from build123d import *

# Parameters (mm, degrees)
F0_W           = 8.4991231561
F0_H           = 6.35
F1_DEPTH       = 12.7
F2_DEPTH       = 16.525
F3_DEPTH       = 7
F5_D           = 3.4544
F5_DEPTH       = 12.7
F5_CSINK_D     = 4.5974
F5_CSINK_ANGLE = 82
F5_TIP         = 1.0378064612


# Not quite as in the source:
# - a length typed as a fraction of an inch, garbled in the dataset ("3 / 203.2 mm" for 3/8 in), is restored


with BuildPart() as f1:
    # F0 (on Right) → F1 (new body)
    with BuildSketch(Plane.YZ):
        with BuildLine():
            ThreePointArc((19.0844833851, -6.525), (17.2246114456, -2.0348719395), (12.7344833851, -0.175))
            Line((12.7344833851, -0.175), (8.4991231561, -0.175))
            Line((8.4991231561, -0.175), (8.4991231561, -6.525))
            Line((8.4991231561, -6.525), (19.0844833851, -6.525))
        make_face()
        with BuildLine():
            Line((-8.4991231561, -0.175), (-12.7344833851, -0.175))
            ThreePointArc((-12.7344833851, -0.175), (-17.2246114456, -2.0348719395), (-19.0844833851, -6.525))
            Line((-19.0844833851, -6.525), (-8.4991231561, -6.525))
            Line((-8.4991231561, -6.525), (-8.4991231561, -0.175))
        make_face()
        with BuildLine():
            ThreePointArc((8.4901041675, 7.0058502143), (0, 3), (-8.4901041675, 7.0058502143))
            Line((-8.4901041675, 7.0058502143), (-12.7344833851, -0.175))
            Line((-12.7344833851, -0.175), (-8.4991231561, -0.175))
            Line((-8.4991231561, -0.175), (0, -0.175))
            Line((0, -0.175), (8.4991231561, -0.175))
            Line((8.4991231561, -0.175), (12.7344833851, -0.175))
            Line((12.7344833851, -0.175), (8.4901041675, 7.0058502143))
        make_face()
        with BuildLine():
            Line((-3.2282481135, 15.9081179517), (-8.4901041675, 7.0058502143))
            ThreePointArc((-8.4901041675, 7.0058502143), (0, 3), (8.4901041675, 7.0058502143))
            Line((8.4901041675, 7.0058502143), (3.2282481135, 15.9081179517))
            ThreePointArc((3.2282481135, 15.9081179517), (3.6172109716, 14.9890828009), (3.75, 14))
            ThreePointArc((3.75, 14), (-0.9890828009, 10.3827890284), (-3.2282481135, 15.9081179517))
        make_face()
        with BuildLine():
            ThreePointArc((3.2282481135, 15.9081179517), (0, 17.75), (-3.2282481135, 15.9081179517))
            ThreePointArc((-3.2282481135, 15.9081179517), (-0.9890828009, 10.3827890284), (3.75, 14))
            ThreePointArc((3.75, 14), (3.6172109716, 14.9890828009), (3.2282481135, 15.9081179517))
        make_face()
        with Locations((4.249561578, -3.35)):
            Rectangle(F0_W, F0_H)
        with Locations((-4.249561578, -3.35)):
            Rectangle(F0_W, F0_H)
    extrude(amount=F1_DEPTH)

    # F0 (on Right) → F2 (join)
    with BuildSketch(Plane.YZ):
        with BuildLine():
            ThreePointArc((3.2282481135, 15.9081179517), (0, 17.75), (-3.2282481135, 15.9081179517))
            ThreePointArc((-3.2282481135, 15.9081179517), (-0.9890828009, 10.3827890284), (3.75, 14))
            ThreePointArc((3.75, 14), (3.6172109716, 14.9890828009), (3.2282481135, 15.9081179517))
        make_face()
    extrude(amount=-F2_DEPTH)

    # F0 (on Right) → F3 (join)
    with BuildSketch(Plane.YZ):
        with BuildLine():
            ThreePointArc((19.0844833851, -6.525), (17.2246114456, -2.0348719395), (12.7344833851, -0.175))
            Line((12.7344833851, -0.175), (8.4991231561, -0.175))
            Line((8.4991231561, -0.175), (8.4991231561, -6.525))
            Line((8.4991231561, -6.525), (19.0844833851, -6.525))
        make_face()
        with BuildLine():
            Line((-8.4991231561, -0.175), (-12.7344833851, -0.175))
            ThreePointArc((-12.7344833851, -0.175), (-17.2246114456, -2.0348719395), (-19.0844833851, -6.525))
            Line((-19.0844833851, -6.525), (-8.4991231561, -6.525))
            Line((-8.4991231561, -6.525), (-8.4991231561, -0.175))
        make_face()
        with Locations((4.249561578, -3.35)):
            Rectangle(F0_W, F0_H)
        with Locations((-4.249561578, -3.35)):
            Rectangle(F0_W, F0_H)
    extrude(amount=-F3_DEPTH)

    # F5
    with Locations(Plane(origin=(0, 0, -6.525), x_dir=(1, 0, 0), z_dir=(0, 0, -1))):
        with Locations((6.35, 0)):
            CounterSinkHole(F5_D / 2, F5_CSINK_D / 2, depth=F5_DEPTH, counter_sink_angle=F5_CSINK_ANGLE)
            with Locations((0, 0, -(F5_DEPTH + F5_TIP / 2))):  # 118° drill point
                Cone(0, F5_D / 2, F5_TIP, mode=Mode.SUBTRACT)


solid = f1.part
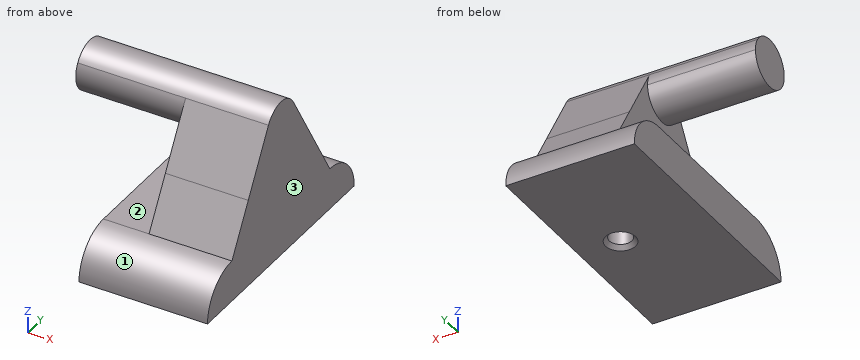
Geometry check sheet. Reference: the model listing, model coordinates, mm. Face numbers are marked on the shaded views. Round coordinates to 2 decimals unless told otherwise and drop trailing zeros. Order: outer loops, then holes, each group sorted by start corner. A loop starts at its lowest first (then second) coordinate and runs counter-clockwise, first axis right, second up. Notation, with made-up numbers: (7.5, 50) - (64.5, 50) arc R21 ccw to (64.5, 89) - close; hole circle Ø1 at (46.25, 88). An arc over 180 degrees is marked (long way). One line per question, with ' | ' between items. Start each with the question number.
(1) Release check for a two-part mould opening along Z. For the marked faces 1, 2 and 3 record: released by +Z, released by -Z, zero draft, split by the parting line, or undercut.
(2) Sectioned sample at B-B on z = 5. Record the cut outline in (x, y).
(3) Sectioned sample at C-C on y = 7.5. Record the cut outline in (x, z) (3 decimals), and give its area (3 significant figures).
(4) Depth check by flat-ended pin: pin 1 Ø1.9 at (y, z) = (-4.5, -2.5) entering from -X; pin 2 Ø5.5 at (x, y) = (-2.5, 5.5) entering from +Z; pin 3 Ø1 at (x, z) = (-11, 12) entering from +Y; pin 4 Ø5 at (x, z) = (-4.5, 6) entering from -Y. Enter the tip coordinate at first touch or a pass-through.
(5) Sectioned sample at A-A on x = 0.5. Record the cut outline in (y, z) (3 decimals).
(6) Thickness scan on L1, parallel to X at y = 6.5, z = 5.5; L2, parallel to X at y = -13, z = -3.75; L3, parallel to Y at x = 7.25, z = -1.25. Record the ranges inside material, lowest first. Write a range as [from, to].
(7) Sectioned sample at D-D on z = 15. Record the cut outline in (x, y) (3 decimals).
Conclusion:
1) face 1: released by +Z | face 2: undercut | face 3: zero draft
2) outline: (0, -9.68) - (12.7, -9.68) - (12.7, 9.68) - (0, 9.68) - close; hole circle Ø3.45 at (6.35, 0)
3) outline: (-7, -6.525) - (12.7, -6.525) - (12.7, 8.681) - (0, 8.681) - (0, -0.175) - (-7, -0.175) - close | area: 238 mm2
4) pin 1: stops at x = -7 | pin 2: stops at z = 16.55 | pin 3: stops at y = 3.44 | pin 4: passes through
5) outline: (-19.084, -6.525) - (19.084, -6.525) arc R6.35 ccw to (12.734, -0.175) - (3.228, 15.908) arc R3.75 ccw to (-3.228, 15.908) - (-12.734, -0.175) arc R6.35 ccw to start
6) L1: x = [0, 12.7] | L2: x = [-7, 12.7] | L3: y = [-16.27, -1.47], [1.47, 16.27]
7) outline: (-16.525, -3.614) - (0, -3.614) - (0, -3.765) - (12.7, -3.765) - (12.7, 3.765) - (0, 3.765) - (0, 3.614) - (-16.525, 3.614) - close
